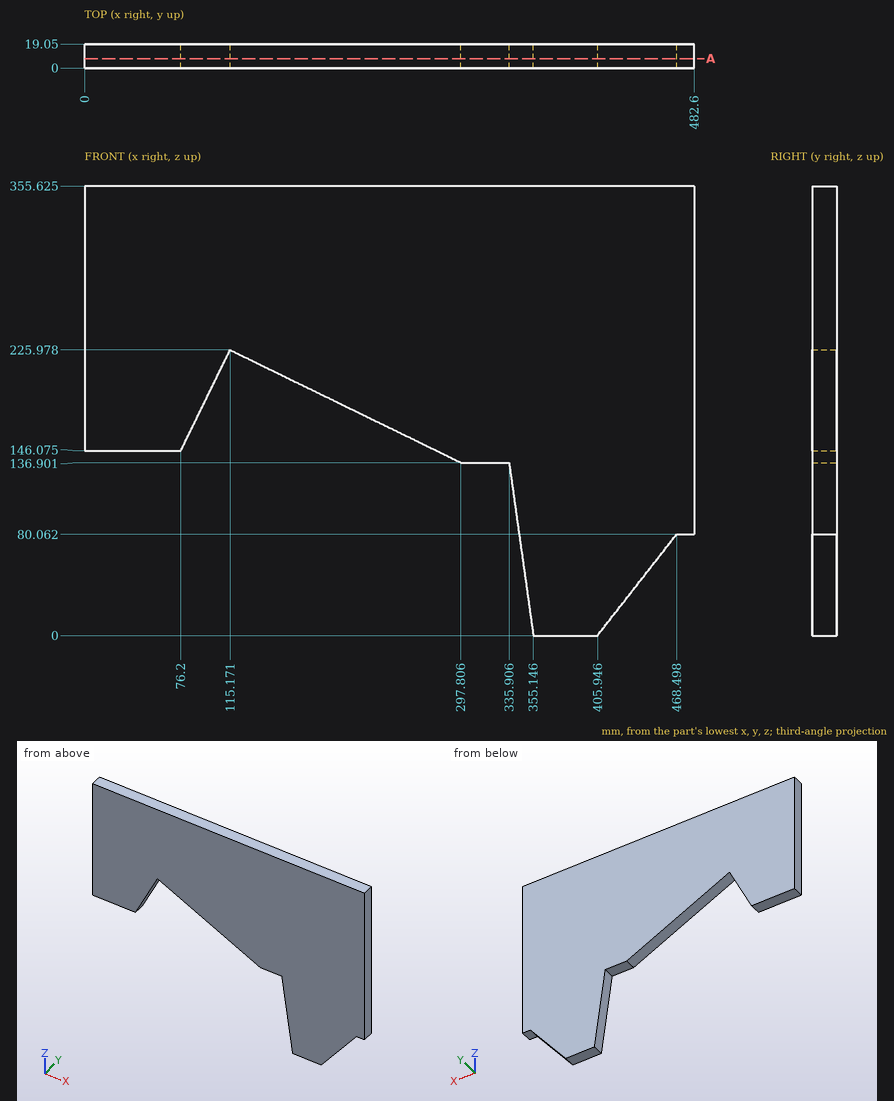
Check sheet for the drawn part. Datum: minimum x, y, z corner. Units: mm. Round coordinates to 2 decimals unless told otherwise and drop trailing zeros. Order: outer loops, then holes, each group sorted by start corner. A loop starts at its lowest first (then second) coordinate and runs counter-clockwise, first axis right, second up. Notation, with made-up numbers: (14.5, 50.25) -> (26.5, 50.25) arc R6 ccw to (26.5, 55.25) -> close; hole circle Ø6 at (-2.75, 84.5). An arc over 180 degrees is marked (long way). Put each result on its own line as item: value. Start each with the question number.
(1) Material ranges on line 1 along X through (y, z) = (9.75, 159) (1 decimal); line 2 along X through (y, z) = (7.75, 206.5) (1 decimal); line 3 along Z through (x, y) = (70.5, 3.25) (1 decimal), recorded low to high.
(2) Section check A-A (y = 7.5). Enter the section's corners in (x, z) (1 decimal).
(3) Depth check by flat-ended pin: pin 1 Ø6 at (y, z) = (17, 45.5) entering from +X; pin 2 Ø10 at (x, y) = (68.5, 9.5) entering from -Z (1 decimal); pin 3 Ø4 at (x, y) = (168, 13.5) entering from -Z. Enter the tip coordinate at first touch or a pass-through.
Completed:
1. line 1: x = 0 to 82.5, 252.5 to 482.6
1. line 2: x = 0 to 105.7, 155.1 to 482.6
1. line 3: z = 146.1 to 355.6
2. outline: (0, 146.1) -> (76.2, 146.1) -> (115.2, 226) -> (297.8, 136.9) -> (335.9, 136.9) -> (355.1, 0) -> (405.9, 0) -> (468.5, 80.1) -> (482.6, 80.1) -> (482.6, 355.6) -> (0, 355.6) -> close
3. pin 1: stops at x = 443.84
3. pin 2: stops at z = 146.1
3. pin 3: stops at z = 199.24
